```python
from build123d import *

# Parameters (mm, degrees)
CROQUIS1_W              = 206
CROQUIS1_H              = 163
SALIENTE_EXTRUIR1_DEPTH = 3
CROQUIS2_W              = 206
CROQUIS2_H              = 163
CROQUIS2_W_2            = 196
CROQUIS2_H_2            = 153
SALIENTE_EXTRUIR2_DEPTH = 3
CROQUIS3_W              = 100
CROQUIS3_H              = 5
CORTAR_EXTRUIR1_DEPTH   = 10
REDONDEO2_R             = 2
CHAFL_N1_SIZE           = 2
CROQUIS4_R              = 1.5
CORTAR_EXTRUIR3_DEPTH   = 10
CROQUIS5_R              = 1.5
CORTAR_EXTRUIR4_DEPTH   = 10


with BuildPart() as part:
    # Croquis1 → Saliente-Extruir1 (new body)
    with BuildSketch(Plane(origin=(0, 0, 0), x_dir=(1, 0, 0), z_dir=(0, 1, 0))):
        with Locations((103, 81.5)):
            Rectangle(CROQUIS1_W, CROQUIS1_H)
    extrude(amount=SALIENTE_EXTRUIR1_DEPTH)

    # Croquis2 → Saliente-Extruir2 (add)
    with BuildSketch(Plane(origin=(0, 3, 0), x_dir=(1, 0, 0), z_dir=(0, 1, 0))):
        with Locations((103, 81.5)):
            Rectangle(CROQUIS2_W, CROQUIS2_H)
        with Locations((103, 81.5)):
            Rectangle(CROQUIS2_W_2, CROQUIS2_H_2, mode=Mode.SUBTRACT)
    extrude(amount=SALIENTE_EXTRUIR2_DEPTH)

    # Croquis3 → Cortar-Extruir1 (cut)
    with BuildSketch(Plane(origin=(0, 6, 0), x_dir=(1, 0, 0), z_dir=(0, 1, 0))):
        with Locations((103, 2.5)):
            Rectangle(CROQUIS3_W, CROQUIS3_H)
    extrude(amount=-CORTAR_EXTRUIR1_DEPTH, mode=Mode.SUBTRACT)

    # Redondeo2
    redondeo2_edges = [part.edges().sort_by_distance(p)[0] for p in [
        (103, 6, -163),
        (26.5, 6, 0),
        (0, 6, -81.5),
        (201, 6, -81.5),
        (103, 6, -158),
        (5, 6, -81.5),
        (206, 6, -81.5),
        (29, 6, -5),
        (177, 6, -5),
        (179.5, 6, 0),
        (53, 6, -2.5),
        (153, 6, -2.5),
    ]]
    fillet(redondeo2_edges, radius=REDONDEO2_R)

    # Chaflán1
    chafl_n1_edges = [part.edges().sort_by_distance(p)[0] for p in [
        (103, 3, -5),
    ]]
    chamfer(chafl_n1_edges, length=CHAFL_N1_SIZE)

    # Croquis4 → Cortar-Extruir3 (cut)
    with BuildSketch(Plane(origin=(0, 3, 0), x_dir=(1, 0, 0), z_dir=(0, 1, 0))):
        with Locations(Location((123, 51.88030089, 0), (0, 0, 270))):
            Circle(CROQUIS4_R)
        with Locations(Location((83, 51.88030089, 0), (0, 0, 270))):
            Circle(CROQUIS4_R)
        with Locations(Location((75, 121.88030089, 0), (0, 0, 270))):
            Circle(CROQUIS4_R)
        with Locations(Location((131, 121.88030089, 0), (0, 0, 270))):
            Circle(CROQUIS4_R)
    extrude(amount=-CORTAR_EXTRUIR3_DEPTH, mode=Mode.SUBTRACT)

    # Croquis5 → Cortar-Extruir4 (cut)
    with BuildSketch(Plane(origin=(0, 3, 0), x_dir=(1, 0, 0), z_dir=(0, 1, 0))):
        with Locations(Location((89, 123, 0), (0, 0, 270))):
            Circle(CROQUIS5_R)
        with Locations(Location((117, 123, 0), (0, 0, 270))):
            Circle(CROQUIS5_R)
        with Locations(Location((89, 83, 0), (0, 0, 270))):
            Circle(CROQUIS5_R)
        with Locations(Location((117, 83, 0), (0, 0, 270))):
            Circle(CROQUIS5_R)
    extrude(amount=-CORTAR_EXTRUIR4_DEPTH, mode=Mode.SUBTRACT)


solid = part.part
```
The model under review builds one solid part; all positions refer to its coordinate system, in mm. A direction names the side the tool comes from. Coordinates: 2 decimals unless noted, no trailing zeros. Write each loop counter-clockwise with the first axis right and the second up, starting at its lowest first coordinate (ties: lowest second). Pieces come first, ordered by that corner, then holes.
1) We need section A-A on z = -10. State the section outline as (x, y) points.
2) To check wall thickness, follow probe 1 along X at (y, z) = (1.2, -83); probe 2 along Z at (x, y) = (117, 1.05); probe 3 along X at (y, z) = (3.05, -53.5). State the ranges of each line that lie inside material, in increasing order.
3) We need section C-C on x = 162. State the section outline as (y, z) points.
4) Machinability: for faces 1 (the face through (153, 2, -3)), 2 (the face through (102, 3, -83)), 3 (the face through (179, 2, 0)), which of the approach directions +Z, -Z, +X, -X, +Y, -Y give a long, thin tool a straight path to every point of the face, cutting with its end or side? Answer none if there is none.
5) The part is to be moulded in two halves that separate along X. For faces 4 (the face through (206, 2, -80)), 5 (the face through (0, 2, -80)), 6 (the face through (53, 2, -3)), say which applies: pulls with the +X half, pulls with the -X half, needs draft (parallel to the pull), parting line crosses it, or undercut.
6) We need section B-B on x = 138. State the section outline as (y, z) points.
7) Clearance check with flat-ended pins moving along their axes: pin 1 Ø0.5 at (x, y) = (91.5, 0.5) entering from +Z; pin 2 Ø2.5 at (x, z) = (89, -123) entering from -Y; pin 3 Ø4 at (x, z) = (117, -83) entering from +Y. State where each tip first meets the part, or that it passes through.
Answer list:
1. outline: (0, 0) - (206, 0) - (206, 4) arc R2 ccw to (204, 6) - (203, 6) arc R2 ccw to (201, 4) - (201, 3) - (5, 3) - (5, 4) arc R2 ccw to (3, 6) - (2, 6) arc R2 ccw to (0, 4) - close
2. probe 1: x = 0 to 87.5, 90.5 to 115.5, 118.5 to 206
2. probe 2: z = -163 to -124.5, -121.5 to -84.5, -81.5 to -5.05
2. probe 3: x = 0 to 5, 201 to 206
3. outline: (0, -163) - (4, -163) arc R2 ccw to (6, -161) - (6, -160) arc R2 ccw to (4, -158) - (3, -158) - (3, -5) - (4, -5) arc R2 ccw to (6, -3) - (6, -2) arc R2 ccw to (4, 0) - (0, 0) - close
4. face 1: +Z, +Y
4. face 2: +Y
4. face 3: +Z, +X, -X, +Y, -Y
5. face 4: pulls with the +X half
5. face 5: pulls with the -X half
5. face 6: undercut
6. outline: (0, -163) - (4, -163) arc R2 ccw to (6, -161) - (6, -160) arc R2 ccw to (4, -158) - (3, -158) - (3, -7) - (1, -5) - (0, -5) - close
7. pin 1: stops at z = -5
7. pin 2: passes through
7. pin 3: stops at y = 3
